Geometry: final body of the model. Coordinates: model frame, mm. A direction names the side the tool comes from. Give positions to 0.01 mm unless a question says otherwise; leave off trailing zeros. Write each loop counter-clockwise with the first axis right and the second up, starting at its lowest first coordinate (ties: lowest second). Pieces come first, ordered by that corner, then holes. Notation, with made-up numbers: M 28,53 L 56,53 A16 cw 56,65 Z; hole C 48,59 d1. An arc over 180 degrees is marked long. Use a Markdown table: item, result. Add a question column.
(1) Material intervals for L1, parallel to Y at x = 0.5, z = 11; L2, parallel to Y at x = -1, z = 0.5, sorted ascending.
(2) Pin query (flat end, axial travel): pin 1 Ø1.5 at (y, z) = (2, 11.5) entering from -X. Return the tip coordinate at first contact, or that it passes through.
(3) Draft query along X for faces 1 (the flat face through (0, 0, 44.45)), 2 (the flat face through (-1.03, 0.6, -1.43)), 3 (the cylindrical face through (0.52, -3.93, -0.23)). Return one class per face: released by +X, released by -X, zero draft, split by the parting line, or undercut.
(4) Reachability of faces 4 (the flat face through (-1, -1, -2.21)), 5 (the cylindrical face through (1.987, -0.626, 21.663)), 6 (the flat face through (0, 0, -0.622)) from +Z, -Z, +X, -X, +Y, -Y: full face, straight path, thin tool, end or side. Return the list, or none.
(5) Cut plane A-A (z = 1). Output: boundary loops of the cut face in (x, y).
Autodesk Inventor part; units mm, degrees
ref_plane "YZ Plane" through (0, 0, 0) normal (1, 0, 0) x (0, 1, 0)
ref_plane "XZ Plane" through (0, 0, 0) normal (0, 1, 0) x (-1, 0, 0)
ref_plane "XY Plane" through (0, 0, 0) normal (0, 0, 1) x (1, 0, 0)
sketch "Sketch1" plane through (0, 0, 0) normal (0, 0, 1) x (1, 0, 0)
  circle A0 centre (0, 0) radius 2.0828
  dimension "d0" = 4.1656
extrude "Extrusion1" add sketch "Sketch1" along normal blind 44.45
sketch "Sketch2" plane through (0, 0, 0) normal (0, 1, 0) x (-1, 0, 0)
  line L0 (0, 0) -> (0, -2.2098)
  line L1 (0, 0) -> (3.9624, 0)
  line L2 (0, -2.2098) -> (2.032, -2.2098)
  line L3 (3.9624, 0) -> (3.9624, 3.6562) construction
  arc A0 (2.032, -2.2098) -> (3.9624, -0.4599) centre (0.1837, 1.7689) ccw
  line L4 (4.5847, 0.6553) -> (4.5847, -0.2608) construction
  line L5 (3.9624, -0.4599) -> (3.9624, 0)
  dimension "d3" = 2.2098
  dimension "d6" = 2.032
  dimension "d19" = 3.9624
revolve "Revolution1" add sketch "Sketch2" angle 360 about axis through (0, 0, 0) along (0, 0, -1)
sketch "Sketch3" plane through (0, 0, -2.2098) normal (0, 0, -1) x (-1, 0, 0)
  circle A0 centre (0, 0) radius 2.032
  line L0 (-0.6874, 1.1906) -> (0.6874, 1.1906)
  line L1 (0.6874, 1.1906) -> (1.3748, 0)
  line L2 (1.3748, 0) -> (0.6874, -1.1906)
  line L3 (0.6874, -1.1906) -> (-0.6874, -1.1906)
  line L4 (-0.6874, -1.1906) -> (-1.3748, 0)
  line L5 (-1.3748, 0) -> (-0.6874, 1.1906)
  dimension "d8" = 2.3813
extrude "Extrusion2" cut sketch "Sketch3" against normal blind 1.5875 contours L0 L1 L2 L3 L4 L5
chamfer "Chamfer1" distance 0.508 angle 45 1 edges at (-2.0828, 0, 44.45)
thread "Thread1"
properties part number "10-32 x500 button head" material "Steel"
Answer list:
| question | item | result |
|---|---|---|
| 1 | L1 | -2.02 to 2.02 |
| 1 | L2 | -1.83 to 1.83 |
| 2 | pin 1 | x = -1.67 |
| 3 | face 1 | zero draft |
| 3 | face 2 | undercut |
| 3 | face 3 | split by the parting line |
| 4 | face 4 | -Z, +X, -X, +Y, -Y |
| 4 | face 5 | +Z |
| 4 | face 6 | -Z |
| 5 | outline | C 0,0 d4.17 |
